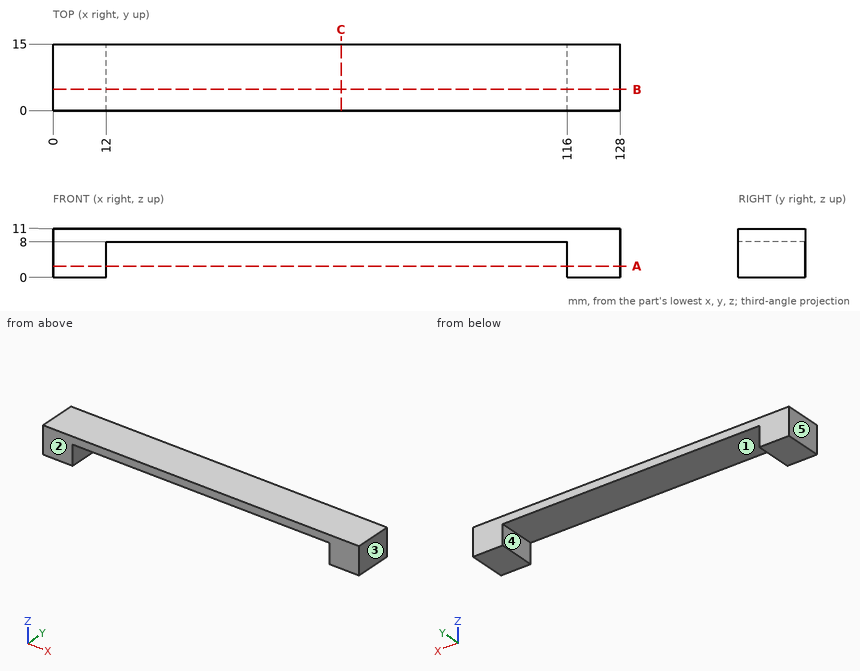
Here's the drawing with two shaded views (mm, measured from the low corner). I have some questions. A direction names the side the tool comes from. Give positions to 0.01 mm unless a question says otherwise; leave off trailing zeros. Loops run counter-clockwise (first coordinate to the right, second up) from the corner with the lowest first, then second, coordinate; pieces in that order, holes last. Notation, with made-up numbers: M -23.5,11 L 6.5,11 A11 cw 6.5,22 Z; hole C -30,11.5 d8. An arc over 180 degrees is marked long. One line per item, written item: value.
(1) Suppose I cut it at C-C on x = 65. List the corners of the cut face in (y, z) for me, plus the area to 3 significant figures.
Returned:
outline: M 0,8 L 15,8 L 15,11 L 0,11 Z
area: 45.0 mm^2
(2) Which directions (+Z, -Z, +X, -X, +Y, -Y) give clear straight access to the entire face, cutting with the end or side of a thin tool? Please do the marked faces 4 and 5.
Returned:
face 4: -Z, +Y, -Y
face 5: +Z, -Z, -X, +Y, -Y
(3) We'd pull the mould along X, two halves only. Please class the marked faces 1, 2 and 3: released by +X, released by -X, zero draft, split by the parting line, or undercut.
Returned:
face 1: undercut
face 2: zero draft
face 3: released by +X
(4) Will this pin go through, and if not, where does the flat tip stop? pin 1 (7.5 mm diameter, centred on x = 85, y = 7, fed in from -Z).
Returned:
pin 1: z = 8
(5) Suppose I cut it at B-B on y = 4.75. List the corners of the cut face in (x, z) for me.
Returned:
outline: M 0,0 L 12,0 L 12,8 L 116,8 L 116,0 L 128,0 L 128,11 L 0,11 Z
(6) I need wall thicknesses on line 1 (X direction, y = 11.75, z = 4); line 2 (Z direction, x = 17, y = 6.5). Which ranges of each line are inside material? Lowest first, please.
Returned:
line 1: 0 to 12, 116 to 128
line 2: 8 to 11
(7) Suppose I cut it at A-A on z = 2.5. List the corners of the cut face in (x, y) for me.
Returned:
outline: M 0,0 L 12,0 L 12,15 L 0,15 Z; M 116,0 L 128,0 L 128,15 L 116,15 Z
